Model file for the job. Use its own axes, mm. Round coordinates to 2 decimals unless told otherwise and drop trailing zeros. Order: outer loops, then holes, each group sorted by start corner. A loop starts at its lowest first (then second) coordinate and runs counter-clockwise, first axis right, second up. Notation, with made-up numbers: (35.5, 1.5) - (52.5, 1.5) arc R36 cw to (52.5, 36.5) - close; hole circle Ø7 at (-16, -12.5). An arc over 180 degrees is marked (long way). Write item = value, one per line.
Autodesk Inventor part; units mm, degrees
ref_plane "YZ Plane" through (0, 0, 0) normal (1, 0, 0) x (0, 1, 0)
ref_plane "XZ Plane" through (0, 0, 0) normal (0, 1, 0) x (-1, 0, 0)
ref_plane "XY Plane" through (0, 0, 0) normal (0, 0, 1) x (1, 0, 0)
sketch "Sketch1" plane through (0, 0, 0) normal (0, 1, 0) x (-1, 0, 0)
  line L0 (49.0311, 150) -> (99.0311, 150)
  line L1 (49.0311, 145) -> (99.0311, 145)
  line L2 (99.0311, 16) -> (49.0311, 16)
  line L3 (99.0311, 11) -> (49.0311, 11)
  line L4 (49.0311, 135) -> (99.0311, 135)
  line L5 (49.0311, 140) -> (99.0311, 140)
  line L6 (99.0311, 43) -> (49.0311, 43)
  line L7 (99.0311, 38) -> (49.0311, 38)
  line L8 (49.0311, 125) -> (99.0311, 125)
  line L9 (99.0311, 70) -> (49.0311, 70)
  line L10 (49.0311, 130) -> (99.0311, 130)
  line L11 (99.0311, 65) -> (49.0311, 65)
  line L12 (49.0311, -11) -> (99.0311, -11)
  line L13 (99.0311, -150) -> (49.0311, -150)
  line L14 (49.0311, -16) -> (99.0311, -16)
  line L15 (99.0311, -145) -> (49.0311, -145)
  line L16 (49.0311, -38) -> (99.0311, -38)
  line L17 (99.0311, -140) -> (49.0311, -140)
  line L18 (49.0311, -43) -> (99.0311, -43)
  line L19 (99.0311, -135) -> (49.0311, -135)
  line L20 (49.0311, -65) -> (99.0311, -65)
  line L21 (49.0311, -70) -> (99.0311, -70)
  line L22 (99.0311, -125) -> (49.0311, -125)
  line L23 (99.0311, -130) -> (49.0311, -130)
  line L24 (99.0311, -160) -> (49.0311, -160)
  line L25 (49.0311, 160) -> (99.0311, 160)
  line L26 (99.0311, -231.4683) -> (49.0311, -231.4683) construction
  line L27 (49.0311, -231.4683) -> (49.0311, 236.8413) construction
  line L28 (49.0311, 236.8413) -> (99.0311, 236.8413) construction
  line L29 (99.0311, 236.8413) -> (99.0311, -231.4683) construction
  line L30 (99.0311, -160) -> (49.0311, -160)
  line L31 (49.0311, -160) -> (49.0311, 160)
  line L32 (49.0311, 160) -> (99.0311, 160)
  line L33 (99.0311, 160) -> (99.0311, -160)
  point P0 (-18.4221, 150)
  dimension "d3" = 5
  dimension "d5" = 5
  dimension "d7" = 5
  dimension "d9" = 5
  dimension "d14" = 5
  dimension "d16" = 5
  dimension "d18" = 5
  dimension "d20" = 22
  dimension "d22" = 5
  dimension "d30" = 5
  dimension "d32" = 5
  dimension "d38" = 5
  dimension "d40" = 5
  dimension "d43" = 5
  dimension "d48" = 5
  dimension "d49" = 5
  dimension "d56" = 10
  dimension "d58" = 10
  dimension "d63" = 50
extrude "Extrusion1" add sketch "Sketch1" along normal blind 10 contours L31 L25 L33 L0 | L1 L33 L5 L31 | L4 L33 L10 L31 | L8 L33 L9 L31 | L11 L33 L6 L31 | L7 L33 L2 L31 | L3 L33 L12 L31 | L14 L33 L16 L31 | L18 L33 L20 L31 | L21 L33 L22 L31 | L23 L33 L19 L31 | L17 L33 L15 L31 | L13 L33 L24 L31
sketch "Sketch2" plane through (0, 10, 0) normal (0, 1, 0) x (1, 0, 0)
  line L0 (-99.0311, 125) -> (-99.0311, 70)
  line L1 (-49.0311, 70) -> (-49.0311, 125)
  line L2 (-99.0311, 122) -> (-49.0311, 122)
  line L3 (-49.0311, 122) -> (-49.0311, 73)
  line L4 (-49.0311, 73) -> (-99.0311, 73)
  line L5 (-99.0311, 73) -> (-99.0311, 122)
  line L6 (-49.0311, 125) -> (-99.0311, 125)
  line L7 (-99.0311, 70) -> (-49.0311, 70)
  line L8 (-99.0311, 65) -> (-99.0311, 43)
  line L9 (-99.0311, 62) -> (-49.0311, 62)
  line L10 (-49.0311, 62) -> (-49.0311, 46)
  line L11 (-49.0311, 46) -> (-99.0311, 46)
  line L12 (-99.0311, 46) -> (-99.0311, 62)
  line L13 (-99.0311, 35) -> (-49.0311, 35)
  line L14 (-49.0311, 35) -> (-49.0311, 19)
  line L15 (-49.0311, 19) -> (-99.0311, 19)
  line L16 (-99.0311, 19) -> (-99.0311, 35)
  line L17 (-49.0311, -11) -> (-49.0311, 11)
  line L18 (-99.0311, 8) -> (-49.0311, 8)
  line L19 (-49.0311, 8) -> (-49.0311, -8)
  line L20 (-49.0311, -8) -> (-99.0311, -8)
  line L21 (-99.0311, -8) -> (-99.0311, 8)
  line L22 (-99.0311, -19) -> (-49.0311, -19)
  line L23 (-49.0311, -19) -> (-49.0311, -35)
  line L24 (-49.0311, -35) -> (-99.0311, -35)
  line L25 (-99.0311, -35) -> (-99.0311, -19)
  line L26 (-99.0311, -43) -> (-99.0311, -65)
  line L27 (-49.0311, -65) -> (-49.0311, -43)
  line L28 (-99.0311, -46) -> (-49.0311, -46)
  line L29 (-49.0311, -46) -> (-49.0311, -62)
  line L30 (-49.0311, -62) -> (-99.0311, -62)
  line L31 (-99.0311, -62) -> (-99.0311, -46)
  line L32 (-49.0311, -125) -> (-49.0311, -70)
  line L33 (-99.0311, -73) -> (-49.0311, -73)
  line L34 (-49.0311, -73) -> (-49.0311, -122)
  line L35 (-49.0311, -122) -> (-99.0311, -122)
  line L36 (-99.0311, -122) -> (-99.0311, -73)
  line L37 (-49.0311, 65) -> (-99.0311, 65)
  line L38 (-99.0311, 43) -> (-49.0311, 43)
  line L39 (-49.0311, 38) -> (-99.0311, 38)
  line L40 (-99.0311, 16) -> (-49.0311, 16)
  line L41 (-49.0311, 11) -> (-99.0311, 11)
  line L42 (-99.0311, -11) -> (-49.0311, -11)
  line L43 (-49.0311, -16) -> (-99.0311, -16)
  line L44 (-99.0311, -38) -> (-49.0311, -38)
  line L45 (-49.0311, -43) -> (-99.0311, -43)
  line L46 (-99.0311, -65) -> (-49.0311, -65)
  line L47 (-49.0311, -70) -> (-99.0311, -70)
  line L48 (-99.0311, -125) -> (-49.0311, -125)
  point P0 (0, 0)
  dimension "d66" = 3
  dimension "d67" = 3
  dimension "d68" = 3
  dimension "d69" = 3
  dimension "d70" = 3
  dimension "d71" = 3
  dimension "d72" = 3
  dimension "d73" = 3
  dimension "d74" = 3
  dimension "d75" = 3
  dimension "d76" = 3
  dimension "d77" = 3
  dimension "d78" = 3
  dimension "d79" = 3
extrude "Extrusion2" cut sketch "Sketch2" against normal blind 10 contours L2 L1 L4 L0 | L9 L10 L11 L8 | L13 L14 L15 L16 | L20 L21 L18 L17 | L22 L23 L24 L25 | L28 L27 L30 L26 | L35 L36 L33 L32
sketch "Sketch3" plane through (-49.0311, 0, -150) normal (1, 0, 0) x (0, 0, -1)
  line L0 (10, 0) -> (10, 10)
  line L1 (10, 0) -> (-310, 0)
  line L2 (-310, 0) -> (-310, -0.5)
  line L3 (-310, -0.5) -> (10, -0.5)
  line L4 (10, -0.5) -> (10, 0)
  point P0 (-150, 0)
  dimension "d82" = 0.5
extrude "Extrusion3" add sketch "Sketch3" against normal blind 50
equation "\"d3\" = d25"
equation "\"d5\" = d26"
equation "\"d7\" = d25"
equation "\"d9\" = d25"
equation "\"d14\" = d25"
equation "\"d16\" = d26"
equation "\"d18\" = d25"
equation "\"d20\" = d28"
equation "\"d22\" = d25"
equation "\"d30\" = d51"
equation "\"d32\" = d51"
equation "\"d38\" = d51"
equation "\"d40\" = d51"
equation "\"d43\" = d51"
equation "\"d48\" = d51"
equation "\"d49\" = d53"
equation "\"d25\" = 5"
equation "\"d26\" = 5"
equation "\"d28\" = -1.2 * d25 + 0.2 * d29"
equation "\"d51\" = 5"
equation "\"d53\" = 5"
equation "\"d54\" = -1.2 * d51 + 0.2 * d55"
properties part number "wire_holder_middle"
1) Cut at A-A (y = 6.25). Give the number of separate pieces and of enclosed holes in the cut face, and give its area (3 significant figures).
Conclusion:
separate_pieces = 20
enclosed_holes = 0
area = 4,100 mm^2
2) Mould opens along Z. For faces 1 (the face through (-74, 5, 160)), 2 (the face through (-74, 5, -135)), 3 (the face through (-74, 10, 155)) say: +Z half, -Z half, draft (parallel to the pull), parting line (faces both ways), or undercut.
Conclusion:
face_1 = +Z half
face_2 = undercut
face_3 = draft
3) Flat gauge pin, fed straight in: pin 1 Ø1.5 at (x, z) = (-82, -136.5) entering from +Y. Where does the tip first touch, or does it go through?
Conclusion:
pin_1 = 0
4) Cut at B-B (z = 56.5). Write the cut outline in (x, y).
Conclusion:
outline = (-99.03, -0.5) - (-49.03, -0.5) - (-49.03, 0) - (-99.03, 0) - close
5) Wall check: line 1 along Y through (x, z) = (-55.5, -42). Give the ranges that are in metal, low to high.
Conclusion:
line_1 = -0.5 to 0
